Can you work these out from the model? Positions are in its coordinate system, mm. Coordinates: 2 decimals unless noted, no trailing zeros.
```python
from build123d import *

# Parameters (mm, degrees)
SKETCH1_R           = 2.1
BOSS_EXTRUDE1_DEPTH = 249.555


with BuildPart() as part:
    # Sketch1 → Boss-Extrude1 (new, symmetric)
    with BuildSketch(Plane(origin=(0, 0, -50), x_dir=(-1, 0, 0), z_dir=(0, 0, -1))):
        with BuildLine():
            Line((10, -7), (10, 7))
            Line((10, 7), (8, 7))
            Line((8, 7), (8, 4))
            Line((8, 4), (7.060660172, 4))
            Line((7.060660172, 4), (4, 7.060660172))
            Line((4, 7.060660172), (4, 9.480384758))
            Line((4, 9.480384758), (3.7, 10))
            Line((3.7, 10), (4, 10.519615242))
            Line((4, 10.519615242), (4, 12.939339828))
            Line((4, 12.939339828), (7.060660172, 16))
            Line((7.060660172, 16), (8, 16))
            Line((8, 16), (8, 13))
            Line((8, 13), (10, 13))
            Line((10, 13), (10, 19))
            ThreePointArc((10, 19), (9.707106781, 19.707106781), (9, 20))
            Line((9, 20), (3, 20))
            Line((3, 20), (3, 18))
            Line((3, 18), (6, 18))
            Line((6, 18), (6, 17.060660172))
            Line((6, 17.060660172), (2.939339828, 14))
            Line((2.939339828, 14), (0.519615242, 14))
            Line((0.519615242, 14), (0, 13.7))
            Line((0, 13.7), (-0.519615242, 14))
            Line((-0.519615242, 14), (-2.939339828, 14))
            Line((-2.939339828, 14), (-6, 17.060660172))
            Line((-6, 17.060660172), (-6, 18))
            Line((-6, 18), (-3, 18))
            Line((-3, 18), (-3, 20))
            Line((-3, 20), (-9, 20))
            ThreePointArc((-9, 20), (-9.707106781, 19.707106781), (-10, 19))
            Line((-10, 19), (-10, 13))
            Line((-10, 13), (-8, 13))
            Line((-8, 13), (-8, 16))
            Line((-8, 16), (-7.060660172, 16))
            Line((-7.060660172, 16), (-4, 12.939339828))
            Line((-4, 12.939339828), (-4, 10.519615242))
            Line((-4, 10.519615242), (-3.7, 10))
            Line((-3.7, 10), (-4, 9.480384758))
            Line((-4, 9.480384758), (-4, 7.060660172))
            Line((-4, 7.060660172), (-7.060660172, 4))
            Line((-7.060660172, 4), (-8, 4))
            Line((-8, 4), (-8, 7))
            Line((-8, 7), (-10, 7))
            Line((-10, 7), (-10, -7))
            Line((-10, -7), (-8, -7))
            Line((-8, -7), (-8, -4))
            Line((-8, -4), (-7.060660172, -4))
            Line((-7.060660172, -4), (-4, -7.060660172))
            Line((-4, -7.060660172), (-4, -9.480384758))
            Line((-4, -9.480384758), (-3.7, -10))
            Line((-3.7, -10), (-4, -10.519615242))
            Line((-4, -10.519615242), (-4, -12.939339828))
            Line((-4, -12.939339828), (-7.060660172, -16))
            Line((-7.060660172, -16), (-8, -16))
            Line((-8, -16), (-8, -13))
            Line((-8, -13), (-10, -13))
            Line((-10, -13), (-10, -19))
            ThreePointArc((-10, -19), (-9.707106781, -19.707106781), (-9, -20))
            Line((-9, -20), (-3, -20))
            Line((-3, -20), (-3, -18))
            Line((-3, -18), (-6, -18))
            Line((-6, -18), (-6, -17.060660172))
            Line((-6, -17.060660172), (-2.939339828, -14))
            Line((-2.939339828, -14), (-0.519615242, -14))
            Line((-0.519615242, -14), (0, -13.7))
            Line((0, -13.7), (0.519615242, -14))
            Line((0.519615242, -14), (2.939339828, -14))
            Line((2.939339828, -14), (6, -17.060660172))
            Line((6, -17.060660172), (6, -18))
            Line((6, -18), (3, -18))
            Line((3, -18), (3, -20))
            Line((3, -20), (9, -20))
            ThreePointArc((9, -20), (9.707106781, -19.707106781), (10, -19))
            Line((10, -19), (10, -13))
            Line((10, -13), (8, -13))
            Line((8, -13), (8, -16))
            Line((8, -16), (7.060660172, -16))
            Line((7.060660172, -16), (4, -12.939339828))
            Line((4, -12.939339828), (4, -10.519615242))
            Line((4, -10.519615242), (3.7, -10))
            Line((3.7, -10), (4, -9.480384758))
            Line((4, -9.480384758), (4, -7.060660172))
            Line((4, -7.060660172), (7.060660172, -4))
            Line((7.060660172, -4), (8, -4))
            Line((8, -4), (8, -7))
            Line((8, -7), (10, -7))
        make_face()
        with Locations(Location((0, -10, 0), (0, 0, 180))):
            Circle(SKETCH1_R, mode=Mode.SUBTRACT)
        with Locations(Location((0, 10, 0), (0, 0, 180))):
            Circle(SKETCH1_R, mode=Mode.SUBTRACT)
        with BuildLine():
            Line((8, 1.7), (8, -1.7))
            ThreePointArc((8, -1.7), (7.912132034, -1.912132034), (7.7, -2))
            Line((7.7, -2), (7.063603897, -2))
            ThreePointArc((7.063603897, -2), (6.948798867, -2.02283614), (6.851471863, -2.087867966))
            Line((6.851471863, -2.087867966), (2.939339828, -6))
            Line((2.939339828, -6), (-2.939339828, -6))
            Line((-2.939339828, -6), (-6.851471863, -2.087867966))
            ThreePointArc((-6.851471863, -2.087867966), (-6.948798867, -2.02283614), (-7.063603897, -2))
            Line((-7.063603897, -2), (-7.7, -2))
            ThreePointArc((-7.7, -2), (-7.912132034, -1.912132034), (-8, -1.7))
            Line((-8, -1.7), (-8, 1.7))
            ThreePointArc((-8, 1.7), (-7.912132034, 1.912132034), (-7.7, 2))
            Line((-7.7, 2), (-7.063603897, 2))
            ThreePointArc((-7.063603897, 2), (-6.948798867, 2.02283614), (-6.851471863, 2.087867966))
            Line((-6.851471863, 2.087867966), (-2.939339828, 6))
            Line((-2.939339828, 6), (2.939339828, 6))
            Line((2.939339828, 6), (6.851471863, 2.087867966))
            ThreePointArc((6.851471863, 2.087867966), (6.948798867, 2.02283614), (7.063603897, 2))
            Line((7.063603897, 2), (7.7, 2))
            ThreePointArc((7.7, 2), (7.912132034, 1.912132034), (8, 1.7))
        make_face(mode=Mode.SUBTRACT)
    extrude(amount=BOSS_EXTRUDE1_DEPTH, both=True)


solid = part.part
```
(1) I want a section at A-A on z = -144.5. State how many separate pieces and enclosed holes the cut face has, then the cut area to 3 significant figures.
Check values:
separate pieces: 1
enclosed holes: 3
area: 324 mm2
(2) If we mould it in two halves opening along X, with no side actions, what happens to faces 1 (the flat face through (10, 0, -53)), 2 (the flat face through (-10, 0, -53)), 3 (the flat face through (5, 5, -299.555))? For each: released by +X, released by -X, zero draft, split by the parting line, or undercut.
Check values:
face 1: released by +X
face 2: released by -X
face 3: zero draft
(3) If I drill on probe 1 along Y at (x, z) = (9, -168); probe 2 along Y at (x, z) = (0, -70); probe 3 along Y at (x, z) = (-7, 27), over which ranges is the centre line in solid material (lowest first)?
Check values:
probe 1: y = -20 to -13, -7 to 7, 13 to 20
probe 2: y = -13.7 to -12.1, -7.9 to -6, 6 to 7.9, 12.1 to 13.7
probe 3: y = -20 to -15.94, -4.06 to -2.01, 2.01 to 4.06, 15.94 to 20
(4) I'm going to push flat-ended pins straight in: pin 1 (5 mm diameter, centred on x = -2.5, z = 2.5, fed in from -Y); pin 2 (0.7 mm diameter, centred on x = 1, z = -137.5, fed in from +Y); pin 3 (1.9 mm diameter, centred on y = 11.5, z = -46.5, fed in from -X). Where does each tip first touch, or does it pass through?
Check values:
pin 1: stops at y = -20
pin 2: stops at y = 14
pin 3: stops at x = -4
